Autodesk Inventor part; units mm, degrees
ref_plane "YZ Plane" through (0, 0, 0) normal (1, 0, 0) x (0, 1, 0)
ref_plane "XZ Plane" through (0, 0, 0) normal (0, 1, 0) x (-1, 0, 0)
ref_plane "XY Plane" through (0, 0, 0) normal (0, 0, 1) x (1, 0, 0)
sketch "Sketch1" plane through (0, 0, 0) normal (0, 1, 0) x (-1, 0, 0)
  line L0 (228.6, 0) -> (228.6, -273.05)
  line L1 (0, -273.05) -> (0, 0)
  line L2 (0, 0) -> (-76.2, 0)
  line L3 (0, 0) -> (-76.2, 0)
  line L4 (228.6, 0) -> (0, 0)
  line L5 (228.6, -273.05) -> (304.8, -273.05)
  line L6 (304.8, -273.05) -> (304.8, -374.65)
  line L7 (304.8, -374.65) -> (-76.2, -374.65)
  line L8 (-76.2, -374.65) -> (-76.2, -273.05)
  line L9 (-76.2, -273.05) -> (0, -273.05)
  line L10 (114.3, -511.2369) -> (114.3, 135.5146) construction
  point P0 (304.8, 0)
  dimension "d1" = 273.05
  dimension "d8" = 228.6
  dimension "d9" = 76.2
  dimension "d10" = 76.2
  dimension "d11" = 101.6
extrude "Extrusion1" add sketch "Sketch1" along normal blind 12.7
sketch "Sketch2" plane through (0, 12.7, 0) normal (0, 1, 0) x (1, 0, 0)
  point P0 (0, 0)
sketch "Sketch3" plane through (0, 12.7, 0) normal (0, 1, 0) x (1, 0, 0)
  line L0 (-114.3, 418.531) -> (-114.3, -18.8119) construction
  circle A0 centre (-241.3, 334.01) radius 14.2875
  line L1 (-304.8, 273.05) -> (-228.6, 273.05) construction
  line L2 (0, 273.05) -> (76.2, 273.05) construction
  circle A1 centre (12.7, 334.01) radius 14.2875
  point P0 (0, 0)
  dimension "d19" = 114.3
  dimension "d20" = 28.575
  dimension "d23" = 60.96
  dimension "d26" = 127
  dimension "d27" = 28.575
  dimension "d28" = 60.96
  dimension "d29" = 127
extrude "Extrusion2" cut sketch "Sketch3" against normal through all
properties part number "shooter bottom" material "Wood (Oak)"
Source: CAD feature listing. Evaluate the final solid. Frame: model axes, mm. A direction names the side the tool comes from. Coordinates: 2 decimals unless noted, no trailing zeros. Order: outer loops, then holes, each group sorted by start corner. A loop starts at its lowest first (then second) coordinate and runs counter-clockwise, first axis right, second up. Notation, with made-up numbers: (-7, 70) - (36, 70) arc R12 cw to (36, 74) - close; hole circle Ø4 at (25, 14.25). An arc over 180 degrees is marked (long way). One line per item, written item: value.
1) Ray query, line 1 (X direction, y = 6.5, z = -334.01); line 2 (Z direction, x = 12.7, y = 10.25); line 3 (X direction, y = 11.5, z = -93). Return the intervals inside material, ascending. Write a range as [from, to].
Computed values:
line 1: x = [-304.8, -255.59], [-227.01, -1.59], [26.99, 76.2]
line 2: z = [-374.65, -348.3], [-319.72, -273.05]
line 3: x = [-228.6, 0]
2) Reachability of faces 4 (the face through (39, 6, -273.05)), 5 (the face through (-112, 0, -226)), 6 (the face through (-228.6, 6, -135)) from +Z, -Z, +X, -X, +Y, -Y: full face, straight path, thin tool, end or side. Return the list, or none.
Computed values:
face 4: +Z, +X, +Y, -Y
face 5: +Z, -Z, +X, -X, -Y
face 6: +Z, -X, +Y, -Y
3) Cut plane D-D on z = -67.5. Output: boundary loops of the cut face in (x, y).
Computed values:
outline: (-228.6, 0) - (0, 0) - (0, 12.7) - (-228.6, 12.7) - close
4) Contact query for a flat-ended pin moving along its axis: pin 1 (2 mm diameter, centred on y = 2, z = -78, fed in from +X). Output: stop coordinate, or through.
Computed values:
pin 1: stops at x = 0
5) Mould query, pull axis X, two halves, no side actions, for faces 1 (the face through (-243.16, 6.439, -348.176)), 2 (the face through (0, 6, -138)), 3 (the face through (-266, 6, -273.05)). Classes: released by +X, released by -X, zero draft, split by the parting line, or undercut.
Computed values:
face 1: undercut
face 2: released by +X
face 3: zero draft
6) Cut plane A-A on x = 12.7. Output: boundary loops of the cut face in (y, z), plus the area to 3 significant figures.
Computed values:
outline: (0, -374.65) - (12.7, -374.65) - (12.7, -348.3) - (0, -348.3) - close; (0, -319.72) - (12.7, -319.72) - (12.7, -273.05) - (0, -273.05) - close
area: 927 mm^2
7) Cut plane B-B on z = -334.01. Output: boundary loops of the cut face in (x, y).
Computed values:
outline: (-304.8, 0) - (-255.59, 0) - (-255.59, 12.7) - (-304.8, 12.7) - close; (-227.01, 0) - (-1.59, 0) - (-1.59, 12.7) - (-227.01, 12.7) - close; (26.99, 0) - (76.2, 0) - (76.2, 12.7) - (26.99, 12.7) - close
8) Cut plane C-C on y = 5.25. State how many separate pieces and enclosed holes the cut face has, plus the area to 3 significant figures.
Computed values:
separate pieces: 1
enclosed holes: 2
area: 99,800 mm^2
